```python
from build123d import *

# Parameters (mm, degrees)
SKETCH2_R           = 2
BOSS_EXTRUDE1_DEPTH = 3


with BuildPart() as part:
    # Sketch2 → Boss-Extrude1 (new body)
    with BuildSketch(Plane(origin=(0, 0, 0), x_dir=(0, 0, -1), z_dir=(1, 0, 0))):
        Polygon((60, 65), (0, 65), (0, 0), (19.65, 0), (19.65, 55), (40.35, 55), (40.35, 0), (60, 0), align=None)
        with Locations((12.5, 60)):
            Circle(SKETCH2_R, mode=Mode.SUBTRACT)
        with Locations((47.5, 60)):
            Circle(SKETCH2_R, mode=Mode.SUBTRACT)
    extrude(amount=BOSS_EXTRUDE1_DEPTH)


solid = part.part
```
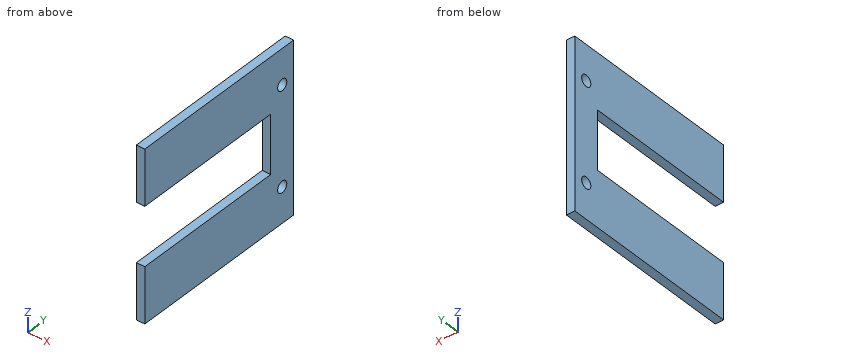
Verification items for the finished model (mm, model axes). Give positions to 0.01 mm unless a question says otherwise; leave off trailing zeros. Order: outer loops, then holes, each group sorted by start corner. A loop starts at its lowest first (then second) coordinate and runs counter-clockwise, first axis right, second up. Notation, with made-up numbers: M 55.5,27 L 108.5,27 A7 ccw 108.5,38 Z; hole C 12.5,39.25 d1. An arc over 180 degrees is marked long. Answer in a Markdown table with one row per item. Add a question column.
Item 1: Section check B-B, the plane y = 9.5. Enter the section's corners in (x, z), and give its area (3 significant figures).
Item 2: Section check A-A, the plane z = -12.5. Enter the section's corners in (x, y), and give its area (3 significant figures).
Item 3: Section check D-D, the plane z = -31.5. Enter the section's corners in (x, y).
Item 4: Section check C-C, the plane x = 1.95. Enter the section's corners in (y, z).
Item 5: Scan lines: probe 1 along Z at (x, y) = (2.1, 34); probe 2 along Y at (x, z) = (1.65, -47.5). Record each from-to range of solid material in increasing order. Write a range as from..to.
Item 6: Gauge pin test, flat ends, axial feed: pin 1 (6 mm diameter, centred on y = 33.5, z = -21, fed in from +X); pin 2 (1.5 mm diameter, centred on x = 1.5, z = -30.5, fed in from -Y). Record the tip position at first contact, or that the pin passes through.
Filled sheet:
| question | item | result |
|---|---|---|
| 1 | outline | M 0,-60 L 3,-60 L 3,-40.35 L 0,-40.35 Z; M 0,-19.65 L 3,-19.65 L 3,0 L 0,0 Z |
| 1 | area | 118 mm^2 |
| 2 | outline | M 0,0 L 3,0 L 3,58 L 0,58 Z; M 0,62 L 3,62 L 3,65 L 0,65 Z |
| 2 | area | 183 mm^2 |
| 3 | outline | M 0,55 L 3,55 L 3,65 L 0,65 Z |
| 4 | outline | M 0,-60 L 65,-60 L 65,0 L 0,0 L 0,-19.65 L 55,-19.65 L 55,-40.35 L 0,-40.35 Z; hole C 60,-47.5 d4; hole C 60,-12.5 d4 |
| 5 | probe 1 | z = -60..-40.35, -19.65..0 |
| 5 | probe 2 | y = 0..58, 62..65 |
| 6 | pin 1 | stops at x = 3 |
| 6 | pin 2 | stops at y = 55 |
